```python
from build123d import *

# Parameters (mm, degrees)
F1_DEPTH = 15
F1_TAPER = 6
F2_R     = 1.8
F3_DEPTH = 15.001
F5_DEPTH = 2.2
F6_R     = 2
F7_R     = 3


with BuildPart() as f1:
    # F0 (on Top) → F1 (new body)
    with BuildSketch(Plane.XY):
        Polygon((-5.7402514855, 5.7402514855), (-8.1179415022, 0), (-5.7402514855, -5.7402514855), (0, -8.1179415022), (5.7402514855, -5.7402514855), (8.1179415022, 0), (5.7402514855, 5.7402514855), (0, 8.1179415022), align=None)
    extrude(amount=F1_DEPTH, taper=F1_TAPER)

    # F2 (on face) → F3 (cut, through all)
    with BuildSketch(Plane.XY.offset(15)):
        Circle(F2_R)
    extrude(amount=-F3_DEPTH, mode=Mode.SUBTRACT)

    # F4 (on face) → F5 (cut)
    with BuildSketch(Plane.XY.offset(15)):
        Polygon((-1.5588457268, 2.7), (-3.1176914536, 0), (-1.5588457268, -2.7), (1.5588457268, -2.7), (3.1176914536, 0), (1.5588457268, 2.7), align=None)
    extrude(amount=-F5_DEPTH, mode=Mode.SUBTRACT)

    # F6
    f6_edges = [f1.edges().sort_by_distance(p)[0] for p in [
        (-5.472542, -2.266801, 15),
        (-2.266801, -5.472542, 15),
        (2.266801, -5.472542, 15),
        (5.472542, -2.266801, 15),
        (5.472542, 2.266801, 15),
        (2.266801, 5.472542, 15),
        (-2.266801, 5.472542, 15),
        (-5.472542, 2.266801, 15),
    ]]
    fillet(f6_edges, radius=F6_R)

    # F7
    f7_edges = [f1.edges().sort_by_distance(p)[0] for p in [
        (-2.870126, -6.929096, 0),
        (-6.929096, -2.870126, 0),
        (2.870126, -6.929096, 0),
        (6.929096, -2.870126, 0),
        (6.929096, 2.870126, 0),
        (2.870126, 6.929096, 0),
        (-2.870126, 6.929096, 0),
        (-6.929096, 2.870126, 0),
    ]]
    fillet(f7_edges, radius=F7_R)


solid = f1.part
```
Verification items for the finished model (mm, model axes). A direction names the side the tool comes from. Give positions to 0.01 mm unless a question says otherwise; leave off trailing zeros. Order: outer loops, then holes, each group sorted by start corner. A loop starts at its lowest first (then second) coordinate and runs counter-clockwise, first axis right, second up. Notation, with made-up numbers: M -7.75,67 L 31.25,67 A36 cw 31.25,103 Z; hole C -2,-4.75 d11. An arc over 180 degrees is marked long. Return JSON: item names as keys, results as strings. Group by question number.
1) Access from +Z, -Z, +X, -X, +Y, -Y to the whole of each face (thin tool, end or side, straight path). Record for faces 5 (the face through (2.35, 1.33, 13.92)), 6 (the face through (1.717, 0.541, 6.49)).
2) Section check B-B on z = 1.75. Record the cut outline in (x, y), and give its area (3 significant figures).
3) Scan lines: line 1 (Z direction, x = -0.75, y = 2.5); line 2 (Y direction, x = 1.5, z = 11.25); line 3 (Y direction, x = 0, z = 7.5). Record each from-to range of solid material in increasing order.
4) Go/stop test with flat-tipped pins: pin 1 Ø1 at (y, z) = (6, 2.5) entering from -X; pin 2 Ø0.7 at (x, z) = (-0.5, 14) entering from +Y; pin 3 Ø1.5 at (x, y) = (3, 5) entering from -Z. Record where each tip stops, or that it passes through.
5) Section check A-A on z = 10.75. Record the cut outline in (x, y).
6) Mould release check, pull along Y, two halves, no side actions. Record for faces 1 (the face through (2.5, 6.15, 8.19)), 2 (the face through (-2.327, 1.369, 13.915)), 3 (the face through (0, 2, 12.8)), 4 (the face through (0, -3, 15)): pulls with the +Y half, pulls with the -Y half, needs draft (parallel to the pull), parting line crosses it, or undercut.
Answer block:
{
 "1": {"face 5": "+Z", "face 6": "+Z, -Z"},
 "2": {"outline": "M -7.46,0 L -5.28,-5.28 L 0,-7.46 L 5.28,-5.28 L 7.46,0 L 5.28,5.28 L 0,7.46 L -5.28,5.28 Z; hole C 0,0 d3.6", "area": "147 mm^2"},
 "3": {"line 1": "z = 0 to 12.8", "line 2": "y = -6.22 to -0.99, 0.99 to 6.22", "line 3": "y = -7.26 to -1.8, 1.8 to 7.26"},
 "4": {"pin 1": "stops at x = -5.36", "pin 2": "stops at y = 6.36", "pin 3": "stops at z = 0.12"},
 "5": {"outline": "M -6.89,0 L -4.88,-4.88 L 0,-6.89 L 4.88,-4.88 L 6.89,0 L 4.88,4.88 L 0,6.89 L -4.88,4.88 Z; hole C 0,0 d3.6"},
 "6": {"face 1": "pulls with the +Y half", "face 2": "undercut", "face 3": "undercut", "face 4": "needs draft"}
}
